```python
from build123d import *

# Parameters (mm, degrees)
SKETCH1_W           = 88.9
SKETCH1_H           = 62.484
BOSS_EXTRUDE1_DEPTH = 5.334
SKETCH2_W           = 17.78
SKETCH2_H           = 14.478
CUT_EXTRUDE1_DEPTH  = 70.229357574
SKETCH3_W           = 9.017
SKETCH3_H           = 5.334
CUT_EXTRUDE2_DEPTH  = 70.229357574
SKETCH5_W           = 5.334
SKETCH5_H           = 12.7
CUT_EXTRUDE3_DEPTH  = 70.229357574
SKETCH7_R           = 1.5
CUT_EXTRUDE4_DEPTH  = 70.229357574


with BuildPart() as part:
    # Sketch1 → Boss-Extrude1 (new body)
    with BuildSketch(Plane.XY):
        with Locations((5.089694656, -16.821198473)):
            Rectangle(SKETCH1_W, SKETCH1_H)
    extrude(amount=BOSS_EXTRUDE1_DEPTH)

    # Sketch2 → Cut-Extrude1 (cut, through all)
    with BuildSketch(Plane.XY.offset(5.334)):
        with Locations((-12.690305344, 7.181801527)):
            Rectangle(SKETCH2_W, SKETCH2_H)
        with Locations((22.869694656, 7.181801527)):
            Rectangle(SKETCH2_W, SKETCH2_H)
    extrude(amount=-CUT_EXTRUDE1_DEPTH, mode=Mode.SUBTRACT)

    # Sketch3 → Cut-Extrude2 (cut, through all)
    with BuildSketch(Plane.XY.offset(5.334)):
        with Locations((-30.406805344, 7.943801527)):
            Rectangle(SKETCH3_W, SKETCH3_H)
        with Locations((5.026194656, 7.943801527)):
            Rectangle(SKETCH3_W, SKETCH3_H)
        with Locations((40.713194656, 7.943801527)):
            Rectangle(SKETCH3_W, SKETCH3_H)
    extrude(amount=-CUT_EXTRUDE2_DEPTH, mode=Mode.SUBTRACT)

    # Sketch5 → Cut-Extrude3 (cut, through all)
    with BuildSketch(Plane.XY.offset(5.334)):
        with Locations((5.089694656, -19.107198473)):
            Rectangle(SKETCH5_W, SKETCH5_H)
    extrude(amount=-CUT_EXTRUDE3_DEPTH, mode=Mode.SUBTRACT)

    # Sketch7 → Cut-Extrude4 (cut, through all)
    with BuildSketch(Plane.XY.offset(5.334)):
        with Locations((-36.225305344, -30.329198473)):
            Circle(SKETCH7_R)
        with Locations((20.924694656, -16.011198473)):
            Circle(SKETCH7_R)
        with Locations((43.924694656, -26.011198473)):
            Circle(SKETCH7_R)
        with Locations((-13.225305344, -20.329198473)):
            Circle(SKETCH7_R)
    extrude(amount=-CUT_EXTRUDE4_DEPTH, mode=Mode.SUBTRACT)


solid = part.part
```
Model file for the job. Use its own axes, mm. A direction names the side the tool comes from. Give positions to 0.01 mm unless a question says otherwise; leave off trailing zeros. Loops run counter-clockwise (first coordinate to the right, second up) from the corner with the lowest first, then second, coordinate; pieces in that order, holes last. Notation, with made-up numbers: (14.25, -4.5) - (65.25, -4.5) arc R16 cw to (65.25, 19.5) - close; hole circle Ø5 at (87.25, -19). An arc over 180 degrees is marked (long way). One line per item, written item: value. Start each with the question number.
1. Which spindle directions (+Z, -Z, +X, -X, +Y, -Y) get a long thin tool onto all of the face, cutting with end or side? Do faces 4 (the flat face through (49.54, -17, 3)), 5 (the flat face through (5, -25.457, 3)), 6 (the flat face through (-21.58, 7, 3)). Say none if no direction does.
2. Slice it at B-B (z = 1.3). Give the number of separate pieces and of enclosed holes in the cut face, plus the area to 3 significant figures.
3. Slice it at A-A (x = -33.5). List the corners of the cut face in (y, z).
4. Probe L1, parallel to X at y = 10, z = 1.95; L2, parallel to X at y = 1.5, z = 0.6; L3, parallel to X at y = -16, z = 2.05. List the from-to ranges inside material, lowest first. Write a range as from..to.
5. Slice it at C-C (x = -16). List the corners of the cut face in (y, z), plus the area to 3 significant figures.
6. Pull direction X, two halves, no side cores. Call faces 1 (the flat face through (36.205, 8, 3)), 2 (the flat face through (-39.36, -17, 3)), 3 (the flat face through (4, -48.063, 3)): pulls with the +X half, pulls with the -X half, needs draft (parallel to the pull), parting line crosses it, or undercut.
Solution:
1. face 4: +Z, -Z, +X, +Y, -Y
1. face 5: +Z, -Z
1. face 6: +Z, -Z, +Y
2. separate pieces: 1
2. enclosed holes: 8
2. area: 4,800 mm^2
3. outline: (-48.06, 0) - (5.28, 0) - (5.28, 5.33) - (-48.06, 5.33) - close; (10.61, 0) - (14.42, 0) - (14.42, 5.33) - (10.61, 5.33) - close
4. L1: x = -39.36..-34.92, -25.9..-21.58, -3.8..0.52, 9.53..13.98, 31.76..36.2, 45.22..49.54
4. L2: x = -39.36..-21.58, -3.8..13.98, 31.76..49.54
4. L3: x = -39.36..2.42, 7.76..19.42, 22.42..49.54
5. outline: (-48.06, 0) - (-0.06, 0) - (-0.06, 5.33) - (-48.06, 5.33) - close
5. area: 256 mm^2
6. face 1: undercut
6. face 2: pulls with the -X half
6. face 3: needs draft
